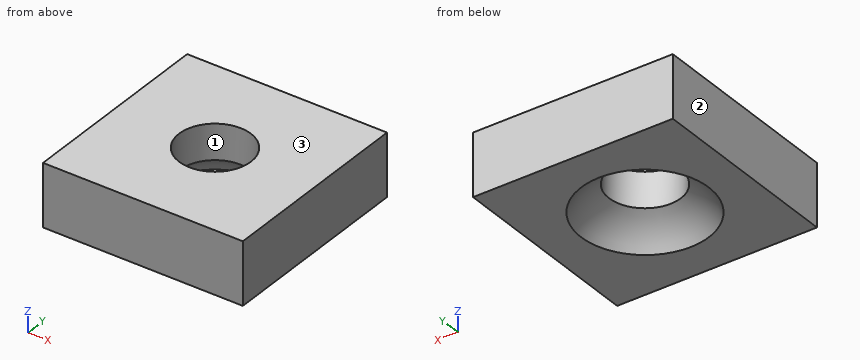
from build123d import *

# Parameters (mm, degrees)
SKETCH3_W      = 15.875
SKETCH3_H      = 50.8
EXTRUDE2_DEPTH = 25.4


with BuildPart() as part:
    # Sketch3 → Extrude2 (new, symmetric)
    with BuildSketch(Plane(origin=(0, 0, 0), x_dir=(0, 0, -1), z_dir=(1, 0, 0))):
        with Locations((-17.4625, 0)):
            Rectangle(SKETCH3_W, SKETCH3_H)
    extrude(amount=EXTRUDE2_DEPTH, both=True)

    # Sketch4 → Cut-Revolve2 (revolve, cut)
    with BuildSketch(Plane(origin=(0, 0, 0), x_dir=(0, 0, -1), z_dir=(1, 0, 0))):
        with BuildLine():
            Line((-34.061608779, 0), (0, 0))
            Line((0, 0), (0, 18.796))
            ThreePointArc((0, 18.796), (-9.531982441, 16.199719959), (-16.430671014, 9.128125))
            Line((-16.430671014, 9.128125), (-34.061608779, 9.128125))
            Line((-34.061608779, 9.128125), (-34.061608779, 0))
        make_face()
    revolve(axis=Axis((0, 0, 0), (0, 0, -1)), mode=Mode.SUBTRACT)


solid = part.part
Read the model definition and answer for the solid it produces. Units are mm, in the model's axes. Face numbers are marked on the shaded views. Coordinates: 2 decimals unless noted, no trailing zeros. Write each loop counter-clockwise with the first axis right and the second up, starting at its lowest first coordinate (ties: lowest second). Pieces come first, ordered by that corner, then holes. Notation, with made-up numbers: (11.25, 50.5) -> (41.25, 50.5) arc R6 ccw to (41.25, 60.5) -> close; hole circle Ø5 at (8.25, 4). An arc over 180 degrees is marked (long way). Return JSON: item names as keys, results as strings.
(1) Consider line 1 along Y through (x, z) = (0, 22.75); line 2 along Y through (x, z) = (-4.5, 20.25). Determine where each line is inside the solid, lowest interval first. Write a range as from..to.
Answers below:
{"line 1": "-25.4..-9.13, 9.13..25.4", "line 2": "-25.4..-7.94, 7.94..25.4"}
(2) The part is cut by section D-D on x = -11. Give the vertices of the cut face in (y, z) (3 decimals), then the cut area to 3 significant figures.
Answers below:
{"outline": "(-25.4, 9.525) -> (-11.898, 9.525) arc R15.241 cw to (11.898, 9.525) -> (25.4, 9.525) -> (25.4, 25.4) -> (-25.4, 25.4) -> close", "area": "712 mm^2"}
(3) The part is cut by section C-C on z = 21.5. Give the vertices of the cut face in (x, y).
Answers below:
{"outline": "(-25.4, -25.4) -> (25.4, -25.4) -> (25.4, 25.4) -> (-25.4, 25.4) -> close; hole circle Ø18.26 at (0, 0)"}
(4) This flat-tipped pin is pushed along its axis until it touches: P1, Ø4, axis at x = 8, y = -9.5, coming from the -Z side. Where does it stop, or does it pass through?
Answers below:
{"P1": "z = 12.06"}
(5) For a pull along X with two mould halves and no side action, classify the marked faces 1, 2 and 3 as pulls with the +X half, pulls with the -X half, needs draft (parallel to the pull), parting line crosses it, or undercut.
Answers below:
{"face 1": "undercut", "face 2": "pulls with the -X half", "face 3": "needs draft"}
(6) The part is cut by section A-A on x = 0. Give the vertices of the cut face in (y, z) (3 decimals), then the cut area to 3 significant figures.
Answers below:
{"outline": "(-25.4, 9.525) -> (-16.204, 9.525) arc R18.796 cw to (-9.128, 16.431) -> (-9.128, 25.4) -> (-25.4, 25.4) -> close; (9.128, 16.431) arc R18.796 cw to (16.204, 9.525) -> (25.4, 9.525) -> (25.4, 25.4) -> (9.128, 25.4) -> close", "area": "459 mm^2"}
